Print and shaded views of the part. All mm, measured from the part's lowest x, y and z. A direction names the side the tool comes from. Round coordinates to 2 decimals unless told otherwise and drop trailing zeros. Order: outer loops, then holes, each group sorted by start corner. A loop starts at its lowest first (then second) coordinate and runs counter-clockwise, first axis right, second up. Notation, with made-up numbers: (76, -38.75) -> (125, -38.75) arc R29 cw to (125, -6.75) -> close; hole circle Ø4 at (-39, 26.25). An arc over 180 degrees is marked (long way). Answer as CSV lines item,"result".
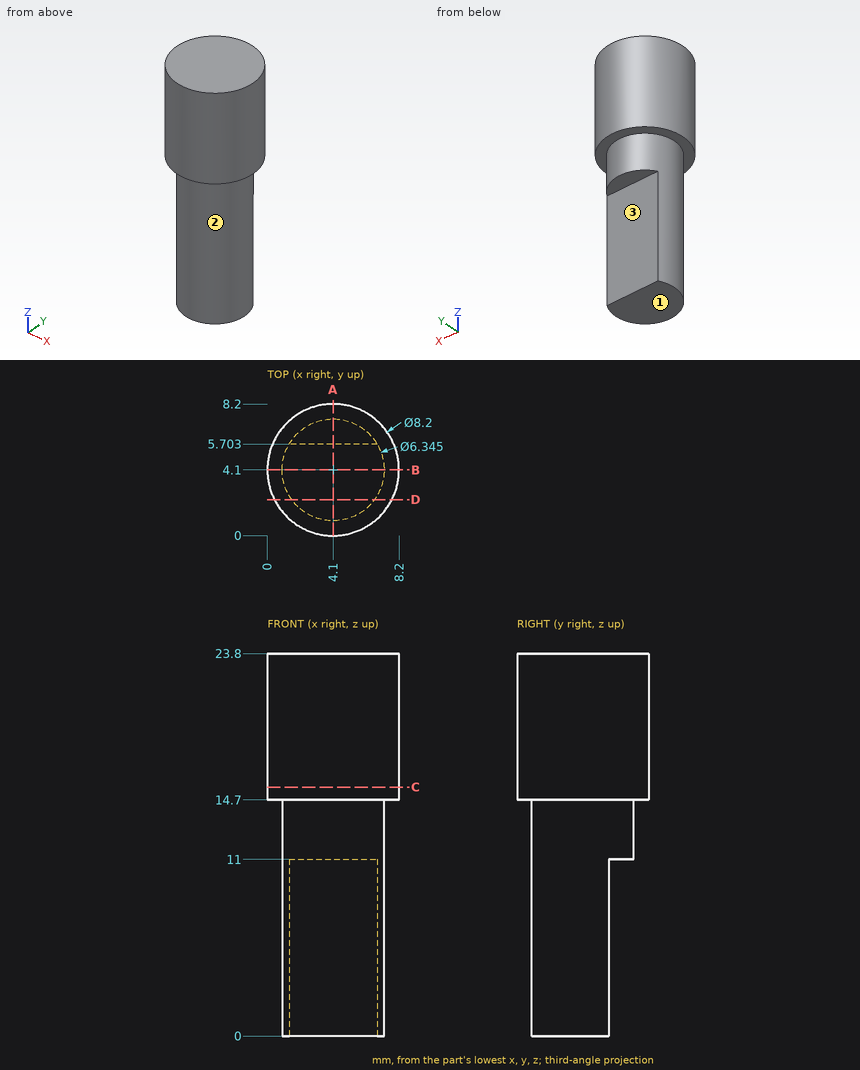
Q1. Saw through at B-B (y = 4.1). Write the cut outline in (x, z).
Checks:
outline,"(0, 14.7) -> (0.93, 14.7) -> (0.93, 0) -> (7.27, 0) -> (7.27, 14.7) -> (8.2, 14.7) -> (8.2, 23.8) -> (0, 23.8) -> close"
Q2. Tool access for the marked faces 1, 2 and 3: list every direction of +Z, -Z, +X, -X, +Y, -Y with a clear straight run to the whole face (end or side of a thin tool).
Checks:
face 1,"-Z, +X, -X, +Y, -Y"
face 2,"-Z"
face 3,"-Z, +X, -X, +Y"
Q3. Saw through at C-C (z = 15.5). Write the cut outline in (x, y), plus the area to 3 significant figures.
Checks:
outline,"circle Ø8.2 at (4.1, 4.1)"
area,"52.8 mm²"
Q4. Saw through at D-D (y = 2.25). Write the cut outline in (x, z).
Checks:
outline,"(0.44, 14.7) -> (1.52, 14.7) -> (1.52, 0) -> (6.68, 0) -> (6.68, 14.7) -> (7.76, 14.7) -> (7.76, 23.8) -> (0.44, 23.8) -> close"
Q5. Saw through at A-A (x = 4.1). Write the cut outline in (y, z).
Checks:
outline,"(0, 14.7) -> (0.93, 14.7) -> (0.93, 0) -> (5.7, 0) -> (5.7, 11) -> (7.27, 11) -> (7.27, 14.7) -> (8.2, 14.7) -> (8.2, 23.8) -> (0, 23.8) -> close"
Q6. Flat gauge pins, fed straight in: pin 1 (2 mm diameter, centred on x = 1, z = 5.5, fed in from -Y); pin 2 (1 mm diameter, centred on y = 7, z = 20, fed in from +X); pin 3 (3 mm diameter, centred on x = 2.5, z = 12, fed in from -Y). Where does each tip first touch, or does it go through?
Checks:
pin 1,"y = 1.72"
pin 2,"x = 7.42"
pin 3,"y = 0.93"
Q7. Wall check: L1, parallel to Y at x = 2.5, z = 4.5; L2, parallel to X at y = 4.25, z = 2.25; L3, parallel to X at y = 2.5, z = 8.75. Give the ranges that are in metal, low to high. Write a range as [from, to].
Checks:
L1,"[1.36, 5.7]"
L2,"[0.93, 7.27]"
L3,"[1.36, 6.84]"
